Verification items for this drawing (mm, ordinates from the low corner). A direction names the side the tool comes from. Coordinates: 2 decimals unless noted, no trailing zeros. Order: outer loops, then holes, each group sorted by start corner. A loop starts at its lowest first (then second) coordinate and runs counter-clockwise, first axis right, second up.
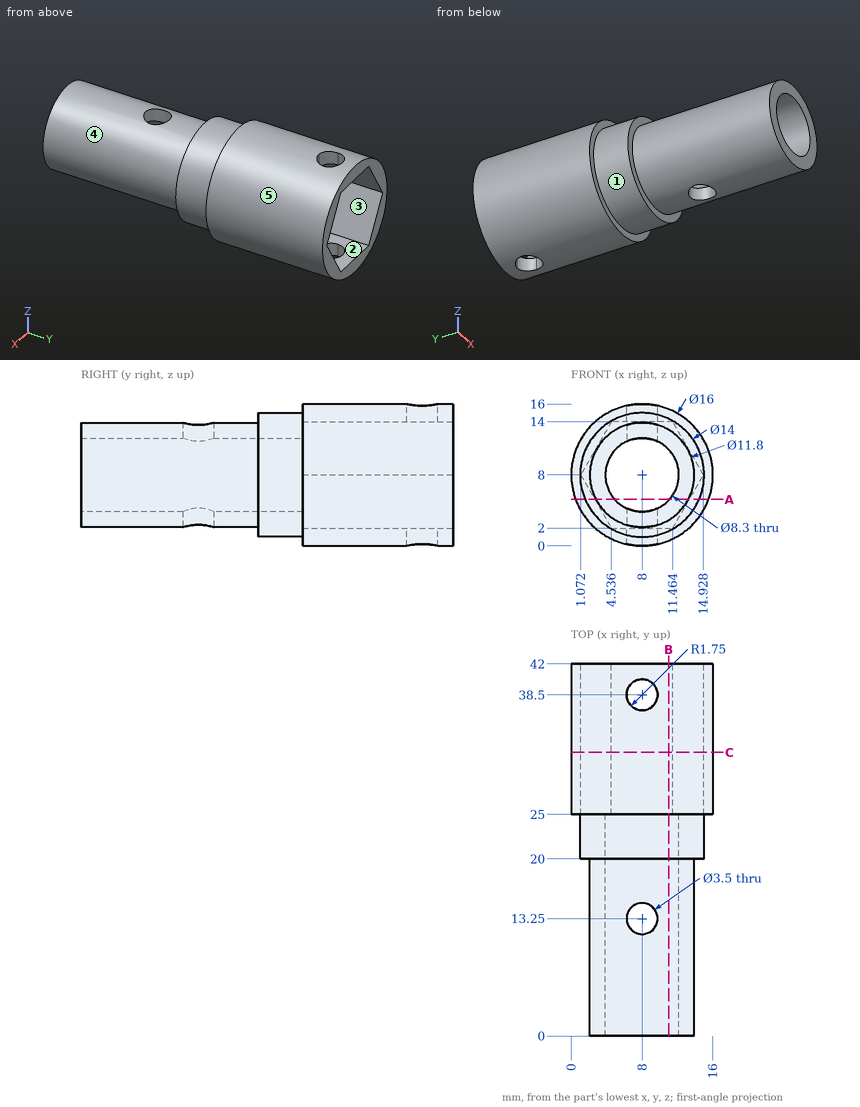
(1) Cross-section at B-B (x = 11). Enter the section's corners in (y, z) (1 decimal).
Filled in:
outline: (0, 2.9) - (20, 2.9) - (20, 1.7) - (25, 1.7) - (25, 0.6) - (42, 0.6) - (42, 2) - (25, 2) - (25, 5.1) - (0, 5.1) - close; (0, 10.9) - (25, 10.9) - (25, 14) - (42, 14) - (42, 15.4) - (25, 15.4) - (25, 14.3) - (20, 14.3) - (20, 13.1) - (0, 13.1) - close
(2) Cross-section at A-A (z = 5.25). Enter the section's corners in (x, y).
Filled in:
outline: (0.49, 25) - (1.56, 25) - (1.56, 20) - (2.78, 20) - (2.78, 0) - (4.89, 0) - (4.89, 25) - (2.66, 25) - (2.66, 42) - (0.49, 42) - close; (11.11, 0) - (13.22, 0) - (13.22, 20) - (14.44, 20) - (14.44, 25) - (15.51, 25) - (15.51, 42) - (13.34, 42) - (13.34, 25) - (11.11, 25) - close
(3) Thickness scan on probe 1 along X at (y, z) = (10.5, 8); probe 2 along Y at (x, z) = (11.25, 13.5); probe 3 along X at (y, z) = (30.5, 3.25) (1 decimal). Record the ranges inside material, lowest first.
Filled in:
probe 1: x = 2.1 to 3.85, 12.15 to 13.9
probe 2: y = 20 to 25
probe 3: x = 1.6 to 3.8, 12.2 to 14.4
(4) Release check for a two-part mould opening along X. For the marked faces 1 and 2 record: +X half, -X half, draft (parallel to the pull), parting line (faces both ways), or undercut.
Filled in:
face 1: parting line
face 2: undercut
(5) Go/stop test with flat-tipped pins: P1, Ø4, axis at y = 10.5, z = 8, coming from the -X side; P2, Ø5, axis at x = 8, z = 8, coming from the -Y side; P3, Ø6, axis at y = 11, z = 13, coming from the +X side; P4, Ø1.5, axis at y = 32.5, z = 2, coming from the +X side (1 decimal). Record where each tip stops, or that it passes through.
Filled in:
P1: stops at x = 2.1
P2: passes through
P3: stops at x = 13.55
P4: stops at x = 14
(6) Cross-section at C-C (y = 32). Enter the section's corners in (x, z).
Filled in:
outline: circle Ø16 at (8, 8); hole (1.07, 8) - (4.54, 2) - (11.46, 2) - (14.93, 8) - (11.46, 14) - (4.54, 14) - close
(7) Tool access check on the marked faces 3, 4 and 5. Record the directions out of +Z, -Z, +X, -X, +Y, -Y that give a thin tool (end or side, any length) a straight path to the whole face; none if there is none.
Filled in:
face 3: +Y
face 4: -Y
face 5: +Y, -Y
